```python
from build123d import *

# Parameters (mm, degrees)
SKETCH1_R           = 25
BOSS_EXTRUDE1_DEPTH = 60
CUT_EXTRUDE1_REACH  = 107
CUT_EXTRUDE1_START  = 45


with BuildPart() as part:
    # Sketch1 → Boss-Extrude1 (new body)
    with BuildSketch(Plane(origin=(0, 0, 0), x_dir=(1, 0, 0), z_dir=(0, 1, 0))):
        Polygon((60.044427996, 0), (30.022213998, 52), (-30.022213998, 52), (-60.044427996, 0), (-30.022213998, -52), (30.022213998, -52), align=None)
        Circle(SKETCH1_R, mode=Mode.SUBTRACT)
    extrude(amount=BOSS_EXTRUDE1_DEPTH)

    # Sketch2 → Cut-Extrude1 (cut, up to next)
    with BuildSketch(Plane(origin=(0, 0, 0), x_dir=(1, 0, 0), z_dir=(0, 1, 0)).offset(CUT_EXTRUDE1_START), mode=Mode.PRIVATE) as cut_extrude1_sk1:
        with BuildLine():
            Line((-47.533320997, -21.669872981), (-42.533320997, -30.330127019))
            Line((-42.533320997, -30.330127019), (-18.713203436, -16.577575733))
            ThreePointArc((-18.713203436, -16.577575733), (-21.650635095, -12.5), (-23.713203436, -7.917321695))
            Line((-23.713203436, -7.917321695), (-47.533320997, -21.669872981))
        make_face()
    cut_extrude1_tool1 = extrude(cut_extrude1_sk1.sketch, amount=CUT_EXTRUDE1_REACH, mode=Mode.PRIVATE) & part.part
    add(cut_extrude1_tool1.solids().sort_by_distance((-33.26901, 45, 19.207872))[0], mode=Mode.SUBTRACT)
    # Sketch2 → Cut-Extrude1 (cut, up to next)
    with BuildSketch(Plane(origin=(0, 0, 0), x_dir=(1, 0, 0), z_dir=(0, 1, 0)).offset(CUT_EXTRUDE1_START), mode=Mode.PRIVATE) as cut_extrude1_sk2:
        with BuildLine():
            Line((-5, -52), (5, -52))
            Line((5, -52), (5, -24.494897428))
            ThreePointArc((5, -24.494897428), (0, -25), (-5, -24.494897428))
            Line((-5, -24.494897428), (-5, -52))
        make_face()
    cut_extrude1_tool2 = extrude(cut_extrude1_sk2.sketch, amount=CUT_EXTRUDE1_REACH, mode=Mode.PRIVATE) & part.part
    add(cut_extrude1_tool2.solids().sort_by_distance((0, 45, 38.415743))[0], mode=Mode.SUBTRACT)
    # Sketch2 → Cut-Extrude1 (cut, up to next)
    with BuildSketch(Plane(origin=(0, 0, 0), x_dir=(1, 0, 0), z_dir=(0, 1, 0)).offset(CUT_EXTRUDE1_START), mode=Mode.PRIVATE) as cut_extrude1_sk3:
        with BuildLine():
            Line((42.533320997, -30.330127019), (47.533320997, -21.669872981))
            Line((47.533320997, -21.669872981), (23.713203436, -7.917321695))
            ThreePointArc((23.713203436, -7.917321695), (21.650635095, -12.5), (18.713203436, -16.577575733))
            Line((18.713203436, -16.577575733), (42.533320997, -30.330127019))
        make_face()
    cut_extrude1_tool3 = extrude(cut_extrude1_sk3.sketch, amount=CUT_EXTRUDE1_REACH, mode=Mode.PRIVATE) & part.part
    add(cut_extrude1_tool3.solids().sort_by_distance((33.26901, 45, 19.207872))[0], mode=Mode.SUBTRACT)
    # Sketch2 → Cut-Extrude1 (cut, up to next)
    with BuildSketch(Plane(origin=(0, 0, 0), x_dir=(1, 0, 0), z_dir=(0, 1, 0)).offset(CUT_EXTRUDE1_START), mode=Mode.PRIVATE) as cut_extrude1_sk4:
        with BuildLine():
            Line((47.533320997, 21.669872981), (42.533320997, 30.330127019))
            Line((42.533320997, 30.330127019), (18.713203436, 16.577575733))
            ThreePointArc((18.713203436, 16.577575733), (21.650635095, 12.5), (23.713203436, 7.917321695))
            Line((23.713203436, 7.917321695), (47.533320997, 21.669872981))
        make_face()
    cut_extrude1_tool4 = extrude(cut_extrude1_sk4.sketch, amount=CUT_EXTRUDE1_REACH, mode=Mode.PRIVATE) & part.part
    add(cut_extrude1_tool4.solids().sort_by_distance((33.26901, 45, -19.207872))[0], mode=Mode.SUBTRACT)
    # Sketch2 → Cut-Extrude1 (cut, up to next)
    with BuildSketch(Plane(origin=(0, 0, 0), x_dir=(1, 0, 0), z_dir=(0, 1, 0)).offset(CUT_EXTRUDE1_START), mode=Mode.PRIVATE) as cut_extrude1_sk5:
        with BuildLine():
            Line((5, 52), (-5, 52))
            Line((-5, 52), (-5, 24.494897428))
            ThreePointArc((-5, 24.494897428), (0, 25), (5, 24.494897428))
            Line((5, 24.494897428), (5, 52))
        make_face()
    cut_extrude1_tool5 = extrude(cut_extrude1_sk5.sketch, amount=CUT_EXTRUDE1_REACH, mode=Mode.PRIVATE) & part.part
    add(cut_extrude1_tool5.solids().sort_by_distance((0, 45, -38.415743))[0], mode=Mode.SUBTRACT)
    # Sketch2 → Cut-Extrude1 (cut, up to next)
    with BuildSketch(Plane(origin=(0, 0, 0), x_dir=(1, 0, 0), z_dir=(0, 1, 0)).offset(CUT_EXTRUDE1_START), mode=Mode.PRIVATE) as cut_extrude1_sk6:
        with BuildLine():
            Line((-42.533320997, 30.330127019), (-47.533320997, 21.669872981))
            Line((-47.533320997, 21.669872981), (-23.713203436, 7.917321695))
            ThreePointArc((-23.713203436, 7.917321695), (-21.650635095, 12.5), (-18.713203436, 16.577575733))
            Line((-18.713203436, 16.577575733), (-42.533320997, 30.330127019))
        make_face()
    cut_extrude1_tool6 = extrude(cut_extrude1_sk6.sketch, amount=CUT_EXTRUDE1_REACH, mode=Mode.PRIVATE) & part.part
    add(cut_extrude1_tool6.solids().sort_by_distance((-33.26901, 45, -19.207872))[0], mode=Mode.SUBTRACT)

    # Sketch3 → Cut-Revolve1 (revolve, cut)
    with BuildSketch(Plane.XY):
        with BuildLine():
            Line((60.044427996, 40), (60.044427996, 60))
            Line((60.044427996, 60), (40.044427996, 60))
            ThreePointArc((40.044427996, 60), (54.186563619, 54.142135624), (60.044427996, 40))
        make_face()
    revolve(axis=Axis((0, 0, 0), (0, -1, 0)), mode=Mode.SUBTRACT)


solid = part.part
```
CAD build for the part. Positions are in the model's coordinates, mm. A direction names the side the tool comes from. Coordinates: 2 decimals unless noted, no trailing zeros. Write each loop counter-clockwise with the first axis right and the second up, starting at its lowest first coordinate (ties: lowest second). Pieces come first, ordered by that corner, then holes. Notation, with made-up numbers: (-39.5, 63.5) -> (-11.5, 63.5) arc R31 cw to (-11.5, 90.5) -> close; hole circle Ø5 at (-7, 35). An arc over 180 degrees is marked (long way). Return JSON: item names as keys, results as strings. Group by question number.
Q1. Drill centre lines: line 1 (Z direction, x = 0, y = 17); line 2 (X direction, y = 20, z = 0); line 3 (Y direction, x = -25.5, z = 12.5). Where is each one in solid material? Low to high.
Q2. Cut at C-C, the plane y = 53. State how many separate pieces and enclosed holes the cut face has, then the cut area to 3 significant figures.
Q3. Flat gauge pins, fed straight in: pin 1 (8 mm diameter, centred on y = 43, z = -20.5, fed in from -X); pin 2 (12 mm diameter, centred on y = 53.5, z = 43, fed in from +X); pin 3 (7.5 mm diameter, centred on y = 50.5, z = -37.5, fed in from -X). Where does each tip first touch, or does it go through?
Q4. Cut at A-A, the plane x = 0. Give the cut face in (y, z).
Q5. Pull direction Z, two halves, no side cores. Call faces 4 (the face through (44.823, 27.535, 26.364)), 5 (the face through (-16, 60, -28)), 6 (the face through (35.46, 52.4, -14.7)): released by +Z, released by -Z, zero draft, split by the parting line, or undercut.
Q6. Cut at B-B, the plane y = 30.5. Give the cut face in (x, z).
Q7. Which spindle directions (+Z, -Z, +X, -X, +Y, -Y) get a long thin tool onto all of the face, cutting with end or side? Do faces 1 (the face through (5, 52, 38)), 2 (the face through (23.846, 29.58, -7.509)), 3 (the face through (-35.46, 52.4, 14.7)). Say none if no direction does.
Returned:
{
 "1": {"line 1": "z = -52 to -25, 25 to 52", "line 2": "x = -60.04 to -25, 25 to 60.04", "line 3": "y = 0 to 45"},
 "2": {"separate pieces": "6", "enclosed holes": "0", "area": "5,510 mm2"},
 "3": {"pin 1": "stops at x = -50.52", "pin 2": "stops at x = 38.68", "pin 3": "stops at x = -40.56"},
 "4": {"outline": "(0, -52) -> (45, -52) -> (45, -25) -> (0, -25) -> close; (0, 25) -> (45, 25) -> (45, 52) -> (0, 52) -> close"},
 "5": {"face 4": "released by +Z", "face 5": "zero draft", "face 6": "undercut"},
 "6": {"outline": "(-60.04, 0) -> (-30.02, -52) -> (30.02, -52) -> (60.04, 0) -> (30.02, 52) -> (-30.02, 52) -> close; hole circle Ø50 at (0, 0)"},
 "7": {"face 1": "+Z, -Z, +Y", "face 2": "+Y, -Y", "face 3": "+Y"}
}
